```python
from build123d import *

# Parameters (mm, degrees)
F0_R     = 10
F0_R_2   = 7.25
F0_R_3   = 5.5
F1_DEPTH = 4
F2_R     = 3
F3_DEPTH = 9.8


with BuildPart() as f1:
    # F0 (on Top) → F1 (new body)
    with BuildSketch(Plane.XY):
        Circle(F0_R)
        Circle(F0_R_2, mode=Mode.SUBTRACT)
        Circle(F0_R_2)
        Circle(F0_R_3, mode=Mode.SUBTRACT)
    extrude(amount=F1_DEPTH)

    # F2
    f2_edges = [f1.edges().sort_by_distance(p)[0] for p in [
        (-10, 0, 4),
    ]]
    fillet(f2_edges, radius=F2_R)

    # F0 (on Top) → F3 (join)
    with BuildSketch(Plane.XY):
        Circle(F0_R_2)
        Circle(F0_R_3, mode=Mode.SUBTRACT)
    extrude(amount=-F3_DEPTH)


solid = f1.part
```
The listing builds one solid part. Answer for the finished solid, in the listing's coordinates (mm). A direction names the side the tool comes from. Coordinates: 2 decimals unless noted, no trailing zeros. Loops run counter-clockwise (first coordinate to the right, second up) from the corner with the lowest first, then second, coordinate; pieces in that order, holes last. Notation, with made-up numbers: (72, -35) - (118, -35) arc R31 ccw to (118, 4) - close; hole circle Ø5 at (42.25, -29). An arc over 180 degrees is marked (long way). Write item = value, one per line.
1) Find the intervals of material crossed by line 1 along Y through (x, z) = (0, -7); line 2 along Y through (x, z) = (-6.75, 1.75); line 3 along Y through (x, z) = (1.25, 2.25), in increasing order.
Responses:
line_1 = -7.25 to -5.5, 5.5 to 7.25
line_2 = -7.25 to 7.25
line_3 = -9.65 to -5.36, 5.36 to 9.65
2) Which of the six approach directions +Z, -Z, +X, -X, +Y, -Y give full straight-line access (tool end or side, diameter ignored) to faces 1 (the face through (3, 5, -9.8)), 2 (the face through (3.35, -6.43, -4.83))?
Responses:
face_1 = -Z, +X, -X, +Y, -Y
face_2 = -Z
3) Each of these flat-tipped pins is pushed along its axis until it touches: P1, Ø5, axis at x = -3.5, z = -1, coming from the +Y side; P2, Ø2, axis at x = -7.5, z = -7, coming from the +Y side; P3, Ø8, axis at x = 4, z = -6.5, coming from the +Y side; P4, Ø10, axis at x = 0, y = 0, coming from the -Z side. Where does it stop, or does it pass through?
Responses:
P1 = 9.93
P2 = 3.21
P3 = 7.25
P4 = through
4) Section C-C (z = -6) is taken. Determine the outline of the cut face in (x, y).
Responses:
outline = circle Ø14.5 at (0, 0); hole circle Ø11 at (0, 0)
5) Section D-D (z = 2.5) is taken. Determine the outline of the cut face in (x, y).
Responses:
outline = circle Ø19.2 at (0, 0); hole circle Ø11 at (0, 0)
6) Section A-A (x = 0) is taken. Determine the outline of the cut face in (y, z).
Responses:
outline = (-10, 0) - (-7.25, 0) - (-7.25, -9.8) - (-5.5, -9.8) - (-5.5, 4) - (-7, 4) arc R3 ccw to (-10, 1) - close; (5.5, -9.8) - (7.25, -9.8) - (7.25, 0) - (10, 0) - (10, 1) arc R3 ccw to (7, 4) - (5.5, 4) - close
